from build123d import *

# Parameters (mm, degrees)
SKETCH1_R           = 5.35
BOSS_EXTRUDE1_DEPTH = 14
SKETCH2_R           = 6.275
BOSS_EXTRUDE2_DEPTH = 2
SKETCH3_R           = 2.85
CUT_EXTRUDE1_DEPTH  = 11.9
SKETCH4_R           = 1
BOSS_EXTRUDE3_DEPTH = 8.9
FILLET1_R           = 1
CHAMFER1_SIZE       = 0.3
SKETCH5_R           = 5.35
SKETCH5_R_2         = 4.6
CUT_EXTRUDE2_DEPTH  = 4
CHAMFER2_SIZE       = 1
SKETCH6_R           = 0.6
SKETCH6_W           = 0.25
SKETCH6_H           = 3
BOSS_EXTRUDE4_DEPTH = 11


with BuildPart() as part:
    # Sketch1 → Boss-Extrude1 (new body)
    with BuildSketch(Plane(origin=(0, 0, 0), x_dir=(1, 0, 0), z_dir=(0, 1, 0))):
        with Locations(Location((0, 0, 0), (0, 0, 270))):
            Circle(SKETCH1_R)
    extrude(amount=BOSS_EXTRUDE1_DEPTH)

    # Sketch2 → Boss-Extrude2 (add)
    with BuildSketch(Plane(origin=(0, 14, 0), x_dir=(1, 0, 0), z_dir=(0, 1, 0))):
        with Locations(Location((0, 0, 0), (0, 0, 270))):
            Circle(SKETCH2_R)
    extrude(amount=BOSS_EXTRUDE2_DEPTH)

    # Sketch3 → Cut-Extrude1 (cut)
    with BuildSketch(Plane(origin=(0, 16, 0), x_dir=(1, 0, 0), z_dir=(0, 1, 0))):
        with Locations(Location((0, 0, 0), (0, 0, 270))):
            Circle(SKETCH3_R)
    extrude(amount=-CUT_EXTRUDE1_DEPTH, mode=Mode.SUBTRACT)

    # Sketch4 → Boss-Extrude3 (add)
    with BuildSketch(Plane(origin=(0, 4.1, 0), x_dir=(1, 0, 0), z_dir=(0, 1, 0))):
        with Locations(Location((0, 0, 0), (0, 0, 270))):
            Circle(SKETCH4_R)
    extrude(amount=BOSS_EXTRUDE3_DEPTH)

    # Fillet1
    fillet1_edges = [part.edges().sort_by_distance(p)[0] for p in [
        (0, 13, -1),
    ]]
    fillet(fillet1_edges, radius=FILLET1_R)

    # Chamfer1
    chamfer1_edges = [part.edges().sort_by_distance(p)[0] for p in [
        (0, 16, -2.85),
        (0, 16, -6.275),
    ]]
    chamfer(chamfer1_edges, length=CHAMFER1_SIZE)

    # Sketch5 → Cut-Extrude2 (cut)
    with BuildSketch(Plane.XZ):
        with Locations(Location((0, 0, 0), (0, 0, 270))):
            Circle(SKETCH5_R)
        with Locations(Location((0, 0, 0), (0, 0, 270))):
            Circle(SKETCH5_R_2, mode=Mode.SUBTRACT)
    extrude(amount=-CUT_EXTRUDE2_DEPTH, mode=Mode.SUBTRACT)

    # Chamfer2
    # the kernel refuses this chamfer: 1 mm, written as the material it takes off along each edge
    with BuildSketch(Plane(origin=(0, 4, 0), x_dir=(0, 0, 1), z_dir=(-1, 0, 0))) as chamfer2_piece_1_section:
        Polygon((5.35, CHAMFER2_SIZE), (5.35 - CHAMFER2_SIZE, 0), (5.35, 0), align=None)
    chamfer2_piece_1 = revolve(axis=Axis((0, 4, 0), (0, 1, 0)), mode=Mode.PRIVATE)
    chamfer2_piece_1 = chamfer2_piece_1 - Plane(origin=(0, 4.621256609, 0), x_dir=(0, 0, -1), z_dir=(0, -1, 0)) * Cylinder(4.6, 22, mode=Mode.PRIVATE)
    add(chamfer2_piece_1, mode=Mode.SUBTRACT)

    # Sketch6 → Boss-Extrude4 (add)
    with BuildSketch(Plane.XZ):
        with Locations(Location((0, 0, 0), (0, 0, 90))):
            Circle(SKETCH6_R)
        with Locations((3.625, 0)):
            Rectangle(SKETCH6_W, SKETCH6_H)
    extrude(amount=BOSS_EXTRUDE4_DEPTH)


solid = part.part
Check sheet for the modelled part. Datum: model origin and axes. Units: mm. A direction names the side the tool comes from. Give positions to 0.01 mm unless a question says otherwise; leave off trailing zeros. Write each loop counter-clockwise with the first axis right and the second up, starting at its lowest first coordinate (ties: lowest second). Pieces come first, ordered by that corner, then holes. Notation, with made-up numbers: (-27.5, -15.75) -> (0.5, -15.75) arc R22 cw to (0.5, 17.25) -> close; hole circle Ø9 at (-22.75, 70). An arc over 180 degrees is marked (long way). Use one line per item in the form item = value. Start each with the question number.
1. Section check C-C (x = 0). Record the cut outline in (y, z) (3 decimals).
2. Access from +Z, -Z, +X, -X, +Y, -Y to the whole of each face (thin tool, end or side, straight path). Record for faces 1 (the cylindrical face through (-1, 8, 0)), 2 (the cylindrical face through (-5.223, 9.437, -1.16)), 3 (the flat face through (-3, 16, 3)).
3. Thickness scan on line 1 along X through (y, z) = (8, 0); line 2 along Y through (x, z) = (2.75, -2.75); line 3 along Y through (x, z) = (-1.25, 1.5). Record the ranges inside material, lowest first. Write a range as from..to.
4. Section check A-A (y = -7.25). Record the cut outline in (x, z).
5. Mould release check, pull along X, two halves, no side actions. Record for faces 4 (the flat face through (3.75, -5, 0)), 5 (the flat face through (0, -11, 0)), 6 (the cylindrical face through (-2.4, 14.8, 5.8)), 7 (the flat face through (3.5, -5, 0)): pulls with the +X half, pulls with the -X half, needs draft (parallel to the pull), parting line crosses it, or undercut.
6. Go/stop test with flat-tipped pins: P1, Ø1, axis at y = 5, z = 0.5, coming from the +X side; P2, Ø1.5, axis at x = 4, y = 6, coming from the -Z side; P3, Ø2, axis at x = -3.5, y = 0.5, coming from the +Z side. Record where each tip stops, or that it passes through.
Conclusion:
q1.outline = (-11, -0.6) -> (0, -0.6) -> (0, -4.6) -> (4.25, -4.6) -> (5, -5.35) -> (14, -5.35) -> (14, -6.275) -> (15.7, -6.275) -> (16, -5.975) -> (16, -3.15) -> (15.7, -2.85) -> (4.1, -2.85) -> (4.1, -1) -> (12, -1) arc R1 ccw to (12, 1) -> (4.1, 1) -> (4.1, 2.85) -> (15.7, 2.85) -> (16, 3.15) -> (16, 5.975) -> (15.7, 6.275) -> (14, 6.275) -> (14, 5.35) -> (5, 5.35) -> (4.25, 4.6) -> (0, 4.6) -> (0, 0.6) -> (-11, 0.6) -> close
q2.face_1 = +Y
q2.face_2 = -Y
q2.face_3 = +Z, -Z, +X, -X, +Y
q3.line_1 = -5.35..-2.85, -1..1, 2.85..5.35
q3.line_2 = 0..16
q3.line_3 = 0..4.1
q4.outline = circle Ø1.2 at (0, 0); (3.5, -1.5) -> (3.75, -1.5) -> (3.75, 1.5) -> (3.5, 1.5) -> close
q5.face_4 = pulls with the +X half
q5.face_5 = needs draft
q5.face_6 = parting line crosses it
q5.face_7 = undercut
q6.P1 = 5.35
q6.P2 = -4.25
q6.P3 = 3.86
